Here's the drawing with two shaded views (mm, measured from the low corner). I have some questions. A direction names the side the tool comes from. Round coordinates to 2 decimals unless told otherwise and drop trailing zeros. Order: outer loops, then holes, each group sorted by start corner. A loop starts at its lowest first (then second) coordinate and runs counter-clockwise, first axis right, second up. Notation, with made-up numbers: (-9, -34) -> (9, -34) arc R7 ccw to (9, -28) -> close; hole circle Ø3 at (-2.5, 77). An arc over 180 degrees is marked (long way). One line per question, with ' | ' between items.
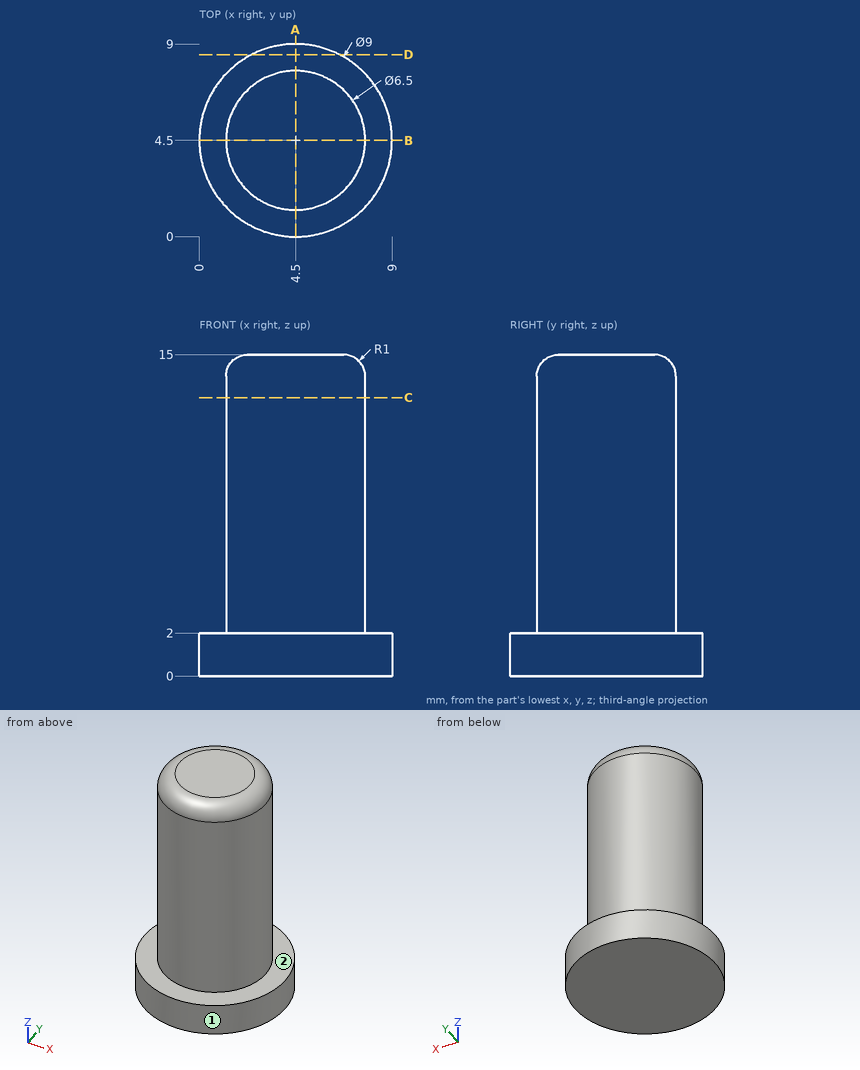
1. I want a section at D-D on y = 8.5. List the corners of the cut face in (x, z) for me, and give its area (3 significant figures).
From the geometry:
outline: (2.44, 0) -> (6.56, 0) -> (6.56, 2) -> (2.44, 2) -> close | area: 8.25 mm²
2. I want a section at C-C on z = 13. List the corners of the cut face in (x, y) for me.
From the geometry:
outline: circle Ø6.5 at (4.5, 4.5)
3. I need wall thicknesses on probe 1 along Z at (x, y) = (1, 3); probe 2 along Z at (x, y) = (5.75, 7); probe 3 along Y at (x, z) = (4, 7.5). Which ranges of each line are inside material? Lowest first, please.
From the geometry:
probe 1: z = 0 to 2 | probe 2: z = 0 to 14.84 | probe 3: y = 1.29 to 7.71
4. On a 3-axis mill with a long thin cutter (end or side, diameter ignored), from which of +Z, -Z, +X, -X, +Y, -Y can I reach the whole of each face in a straight line? I mean the marked faces 1 and 2. Say none if no direction works.
From the geometry:
face 1: +Z, -Z | face 2: +Z
5. I want a section at A-A on x = 4.5. List the corners of the cut face in (y, z) for me.
From the geometry:
outline: (0, 0) -> (9, 0) -> (9, 2) -> (7.75, 2) -> (7.75, 14) arc R1 ccw to (6.75, 15) -> (2.25, 15) arc R1 ccw to (1.25, 14) -> (1.25, 2) -> (0, 2) -> close
6. I'm going to push flat-ended pins straight in: pin 1 (1 mm diameter, centred on y = 3.5, z = 9.5, fed in from -X); pin 2 (5 mm diameter, centred on x = 1, z = 3.5, fed in from -Y). Where does each tip first touch, or does it pass through?
From the geometry:
pin 1: stops at x = 1.29 | pin 2: stops at y = 0.26
